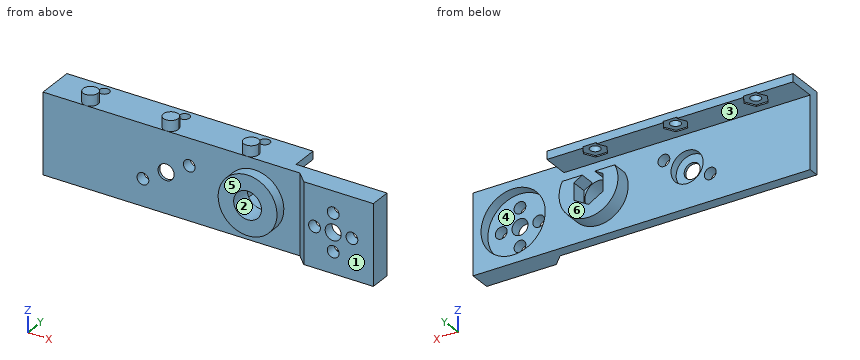
```python
from build123d import *

# Parameters (mm, degrees)
SKETCH_1_W          = 63
SKETCH_1_H          = 15
SKETCH_1_R          = 1.1
SKETCH_1_R_2        = 1.5
SKETCH_1_R_3        = 2.6
EXTRUDE_1_DEPTH     = 2
EXTRUDE_2_DEPTH     = 2
SKETCH_4_R          = 3
CUT_EXTRUDE_1_DEPTH = 1.5
SKETCH_5_W          = 46
SKETCH_5_H          = 1.5
EXTRUDE_3_DEPTH     = 5
SKETCH_2_3_R        = 0.95
CUT_EXTRUDE_2_DEPTH = 6
CUT_EXTRUDE_START   = -0.25
SKETCH_7_R          = 0.95
CUT_EXTRUDE_3_DEPTH = 0.25
SKETCH_1_3_W        = 15
SKETCH_1_3_H        = 15
SKETCH_1_3_R        = 6
SKETCH_1_3_R_2      = 1.5
SKETCH_1_3_R_3      = 1.1
EXTRUDE_4_DEPTH     = 2
EXTRUDE_START       = -2
SKETCH_1_4_W        = 15
SKETCH_1_4_H        = 15
SKETCH_1_4_R        = 6
SKETCH_1_4_R_2      = 1.5
SKETCH_1_4_R_3      = 1.1
EXTRUDE_5_DEPTH     = 2
SKETCH_1_5_R        = 6
CUT_EXTRUDE_4_DEPTH = 2
CUT_EXTRUDE_5_DEPTH = 15
SKETCH_9_R          = 5.5
SKETCH_9_R_2        = 2.6
EXTRUDE_6_DEPTH     = 3
CUT_EXTRUDE_START_2 = -3
CUT_EXTRUDE_6_DEPTH = 3
CUT_EXTRUDE_START_3 = -3.5
CUT_EXTRUDE_7_DEPTH = 3.5
EXTRUDE_START_2     = -4
SKETCH_9_2_R        = 5.5
SKETCH_9_2_R_2      = 2.6
EXTRUDE_7_DEPTH     = 4


with BuildPart() as part:
    # 草图1 → 凸台-拉伸1 (new body)
    with BuildSketch(Plane(origin=(0, 0, 0), x_dir=(1, 0, 0), z_dir=(0, 1, 0))):
        Rectangle(SKETCH_1_W, SKETCH_1_H)
        with Locations(Location((-4.169872981, -2.5, 0), (0, 0, 270))):
            Circle(SKETCH_1_R, mode=Mode.SUBTRACT)
        with Locations(Location((-8.5, 0, 0), (0, 0, 270))):
            Circle(SKETCH_1_R_2, mode=Mode.SUBTRACT)
        with Locations(Location((-12.830127019, 2.5, 0), (0, 0, 270))):
            Circle(SKETCH_1_R, mode=Mode.SUBTRACT)
        with Locations(Location((8, 0, 0), (0, 0, 270))):
            Circle(SKETCH_1_R_3, mode=Mode.SUBTRACT)
        with Locations(Location((24, 3.5, 0), (0, 0, 270))):
            Circle(SKETCH_1_R, mode=Mode.SUBTRACT)
        with Locations(Location((24, -3.5, 0), (0, 0, 270))):
            Circle(SKETCH_1_R, mode=Mode.SUBTRACT)
        with Locations(Location((20.5, 0, 0), (0, 0, 270))):
            Circle(SKETCH_1_R, mode=Mode.SUBTRACT)
        with Locations(Location((24, 0, 0), (0, 0, 270))):
            Circle(SKETCH_1_R_2, mode=Mode.SUBTRACT)
        with Locations(Location((27.5, 0, 0), (0, 0, 270))):
            Circle(SKETCH_1_R, mode=Mode.SUBTRACT)
    extrude(amount=EXTRUDE_1_DEPTH)

    # 草图2 → 凸台-拉伸2 (add)
    with BuildSketch(Plane.XY.offset(7.5)):
        with BuildLine():
            Line((-22.1, 1.4), (-24.9, 1.4))
            ThreePointArc((-24.9, 1.4), (-23.5, 0), (-22.1, 1.4))
        make_face()
        with BuildLine():
            ThreePointArc((-24.764911064, 2), (-24.865810289, 1.707509764), (-24.9, 1.4))
            Line((-24.9, 1.4), (-22.1, 1.4))
            ThreePointArc((-22.1, 1.4), (-22.134189711, 1.707509764), (-22.235088936, 2))
            Line((-22.235088936, 2), (-24.764911064, 2))
        make_face()
        with BuildLine():
            ThreePointArc((-22.235088936, 2), (-23.5, 2.8), (-24.764911064, 2))
            Line((-24.764911064, 2), (-22.235088936, 2))
        make_face()
        with BuildLine():
            Line((-7.1, 1.4), (-9.9, 1.4))
            ThreePointArc((-9.9, 1.4), (-8.5, 0), (-7.1, 1.4))
        make_face()
        with BuildLine():
            ThreePointArc((-9.764911064, 2), (-9.865810289, 1.707509764), (-9.9, 1.4))
            Line((-9.9, 1.4), (-7.1, 1.4))
            ThreePointArc((-7.1, 1.4), (-7.134189711, 1.707509764), (-7.235088936, 2))
            Line((-7.235088936, 2), (-9.764911064, 2))
        make_face()
        with BuildLine():
            ThreePointArc((-7.235088936, 2), (-8.5, 2.8), (-9.764911064, 2))
            Line((-9.764911064, 2), (-7.235088936, 2))
        make_face()
        with BuildLine():
            Line((7.9, 1.4), (5.1, 1.4))
            ThreePointArc((5.1, 1.4), (6.5, 0), (7.9, 1.4))
        make_face()
        with BuildLine():
            ThreePointArc((5.235088936, 2), (5.134189711, 1.707509764), (5.1, 1.4))
            Line((5.1, 1.4), (7.9, 1.4))
            ThreePointArc((7.9, 1.4), (7.865810289, 1.707509764), (7.764911064, 2))
            Line((7.764911064, 2), (5.235088936, 2))
        make_face()
        with BuildLine():
            ThreePointArc((7.764911064, 2), (6.5, 2.8), (5.235088936, 2))
            Line((5.235088936, 2), (7.764911064, 2))
        make_face()
    extrude(amount=EXTRUDE_2_DEPTH)

    # 草图4 → 切除-拉伸1 (cut)
    with BuildSketch(Plane(origin=(0, 2, 0), x_dir=(1, 0, 0), z_dir=(0, 1, 0))):
        with Locations(Location((-8.5, 0, 0), (0, 0, 270))):
            Circle(SKETCH_4_R)
    extrude(amount=-CUT_EXTRUDE_1_DEPTH, mode=Mode.SUBTRACT)

    # 草图5 → 凸台-拉伸3 (add)
    with BuildSketch(Plane(origin=(0, 2, 0), x_dir=(1, 0, 0), z_dir=(0, 1, 0))):
        with Locations((-8.5, -6.75)):
            Rectangle(SKETCH_5_W, SKETCH_5_H)
    extrude(amount=EXTRUDE_3_DEPTH)

    # 草图2<3> → 切除-拉伸2 (cut)
    with BuildSketch(Plane.XY.offset(7.5)):
        with Locations((-23.5, 5.4)):
            Circle(SKETCH_2_3_R)
        with Locations((-8.5, 5.4)):
            Circle(SKETCH_2_3_R)
        with Locations((6.5, 5.4)):
            Circle(SKETCH_2_3_R)
    extrude(amount=-CUT_EXTRUDE_2_DEPTH, mode=Mode.SUBTRACT)

    # 草图7 → 切除-拉伸3 (cut)
    # profile 1 of 3: a face of its own
    with BuildSketch(Plane(origin=(0, 0, 6), x_dir=(-1, 0, 0), z_dir=(0, 0, -1)).offset(CUT_EXTRUDE_START)):
        Polygon((-7.596965511, 3.5), (-5.403034489, 3.5), (-4.306068977, 5.4), (-5.403034489, 7.3), (-7.596965511, 7.3), (-8.693931023, 5.4), align=None)
        with Locations(Location((-6.5, 5.4, 0), (0, 0, 180))):
            Circle(SKETCH_7_R, mode=Mode.SUBTRACT)
    # profile 2 of 3: a face of its own
    with BuildSketch(Plane(origin=(0, 0, 6), x_dir=(-1, 0, 0), z_dir=(0, 0, -1)).offset(CUT_EXTRUDE_START)):
        Polygon((6.306068977, 5.4), (7.403034489, 3.5), (9.596965511, 3.5), (10.693931023, 5.4), (9.596965511, 7.3), (7.403034489, 7.3), align=None)
        with Locations(Location((8.5, 5.4, 0), (0, 0, 180))):
            Circle(SKETCH_7_R, mode=Mode.SUBTRACT)
    # profile 3 of 3: a face of its own
    with BuildSketch(Plane(origin=(0, 0, 6), x_dir=(-1, 0, 0), z_dir=(0, 0, -1)).offset(CUT_EXTRUDE_START)):
        Polygon((21.306068977, 5.4), (22.403034489, 3.5), (24.596965511, 3.5), (25.693931023, 5.4), (24.596965511, 7.3), (22.403034489, 7.3), align=None)
    extrude(amount=CUT_EXTRUDE_3_DEPTH, mode=Mode.SUBTRACT)

    # 草图1<3> → 凸台-拉伸4 (add)
    # profile 1 of 2: a face of its own
    with BuildSketch(Plane(origin=(0, 0, 0), x_dir=(1, 0, 0), z_dir=(0, 1, 0))):
        with Locations((24, 0)):
            Rectangle(SKETCH_1_3_W, SKETCH_1_3_H)
        with Locations((24, 0)):
            Circle(SKETCH_1_3_R, mode=Mode.SUBTRACT)
    # profile 2 of 2: a face of its own
    with BuildSketch(Plane(origin=(0, 0, 0), x_dir=(1, 0, 0), z_dir=(0, 1, 0))):
        with Locations((24, 0)):
            Circle(SKETCH_1_3_R)
        with Locations(Location((24, 0, 0), (0, 0, 270))):
            Circle(SKETCH_1_3_R_2, mode=Mode.SUBTRACT)
        with Locations(Location((27.5, 0, 0), (0, 0, 270))):
            Circle(SKETCH_1_3_R_3, mode=Mode.SUBTRACT)
        with Locations(Location((24, -3.5, 0), (0, 0, 270))):
            Circle(SKETCH_1_3_R_3, mode=Mode.SUBTRACT)
        with Locations(Location((20.5, 0, 0), (0, 0, 270))):
            Circle(SKETCH_1_3_R_3, mode=Mode.SUBTRACT)
        with Locations(Location((24, 3.5, 0), (0, 0, 270))):
            Circle(SKETCH_1_3_R_3, mode=Mode.SUBTRACT)
    extrude(amount=EXTRUDE_4_DEPTH)

    # 草图1<4> → 凸台-拉伸5 (add)
    # profile 1 of 2: a face of its own
    with BuildSketch(Plane(origin=(0, 0, 0), x_dir=(1, 0, 0), z_dir=(0, 1, 0)).offset(EXTRUDE_START)):
        with Locations((24, 0)):
            Rectangle(SKETCH_1_4_W, SKETCH_1_4_H)
        with Locations((24, 0)):
            Circle(SKETCH_1_4_R, mode=Mode.SUBTRACT)
    # profile 2 of 2: a face of its own
    with BuildSketch(Plane(origin=(0, 0, 0), x_dir=(1, 0, 0), z_dir=(0, 1, 0)).offset(EXTRUDE_START)):
        with Locations((24, 0)):
            Circle(SKETCH_1_4_R)
        with Locations(Location((24, 0, 0), (0, 0, 270))):
            Circle(SKETCH_1_4_R_2, mode=Mode.SUBTRACT)
        with Locations(Location((27.5, 0, 0), (0, 0, 270))):
            Circle(SKETCH_1_4_R_3, mode=Mode.SUBTRACT)
        with Locations(Location((24, -3.5, 0), (0, 0, 270))):
            Circle(SKETCH_1_4_R_3, mode=Mode.SUBTRACT)
        with Locations(Location((20.5, 0, 0), (0, 0, 270))):
            Circle(SKETCH_1_4_R_3, mode=Mode.SUBTRACT)
        with Locations(Location((24, 3.5, 0), (0, 0, 270))):
            Circle(SKETCH_1_4_R_3, mode=Mode.SUBTRACT)
    extrude(amount=EXTRUDE_5_DEPTH)

    # 草图1<5> → 切除-拉伸4 (cut)
    with BuildSketch(Plane(origin=(0, 0, 0), x_dir=(1, 0, 0), z_dir=(0, 1, 0))):
        with Locations(Location((24, 0, 0), (0, 0, 270))):
            Circle(SKETCH_1_5_R)
    extrude(amount=CUT_EXTRUDE_4_DEPTH, mode=Mode.SUBTRACT)

    # 草图8 → 切除-拉伸5 (cut)
    with BuildSketch(Plane(origin=(0, 0, -7.5), x_dir=(-1, 0, 0), z_dir=(0, 0, -1))):
        Polygon((-16.5, 0), (-18.5, -2), (-16.5, -2), align=None)
    extrude(amount=-CUT_EXTRUDE_5_DEPTH, mode=Mode.SUBTRACT)

    # 草图9 → 凸台-拉伸6 (add)
    with BuildSketch(Plane(origin=(0, 2, 0), x_dir=(1, 0, 0), z_dir=(0, 1, 0))):
        with Locations(Location((8, 0, 0), (0, 0, 270))):
            Circle(SKETCH_9_R)
        with Locations(Location((8, 0, 0), (0, 0, 270))):
            Circle(SKETCH_9_R_2, mode=Mode.SUBTRACT)
    extrude(amount=EXTRUDE_6_DEPTH)

    # 草图10 → 切除-拉伸6 (cut)
    with BuildSketch(Plane(origin=(0, 5, 0), x_dir=(1, 0, 0), z_dir=(0, 1, 0)).offset(CUT_EXTRUDE_START_2)):
        with BuildLine():
            Line((8, -3.175426481), (6.830127019, -2.5))
            Line((6.830127019, -2.5), (3.101020514, -2.5))
            ThreePointArc((3.101020514, -2.5), (8, -5.5), (12.898979486, -2.5))
            Line((12.898979486, -2.5), (9.169872981, -2.5))
            Line((9.169872981, -2.5), (8, -3.175426481))
        make_face()
        with BuildLine():
            Line((7.285857157, -2.5), (6.830127019, -2.5))
            Line((6.830127019, -2.5), (8, -3.175426481))
            Line((8, -3.175426481), (9.169872981, -2.5))
            Line((9.169872981, -2.5), (8.714142843, -2.5))
            ThreePointArc((8.714142843, -2.5), (8, -2.6), (7.285857157, -2.5))
        make_face()
    extrude(amount=CUT_EXTRUDE_6_DEPTH, mode=Mode.SUBTRACT)

    # 草图10<3> → 切除-拉伸7 (cut)
    with BuildSketch(Plane(origin=(0, 5, 0), x_dir=(1, 0, 0), z_dir=(0, 1, 0)).offset(CUT_EXTRUDE_START_3)):
        with BuildLine():
            Line((10.75, 1.58771324), (8, 3.175426481))
            Line((8, 3.175426481), (5.25, 1.58771324))
            Line((5.25, 1.58771324), (5.25, -1.58771324))
            Line((5.25, -1.58771324), (6.830127019, -2.5))
            Line((6.830127019, -2.5), (7.285857157, -2.5))
            ThreePointArc((7.285857157, -2.5), (6.43423683, 2.075665121), (10.6, 0))
            ThreePointArc((10.6, 0), (10.075665121, -1.56576317), (8.714142843, -2.5))
            Line((8.714142843, -2.5), (9.169872981, -2.5))
            Line((9.169872981, -2.5), (10.75, -1.58771324))
            Line((10.75, -1.58771324), (10.75, 1.58771324))
        make_face()
    extrude(amount=CUT_EXTRUDE_7_DEPTH, mode=Mode.SUBTRACT)

    # 草图9<2> → 凸台-拉伸7 (add)
    with BuildSketch(Plane(origin=(0, 2, 0), x_dir=(1, 0, 0), z_dir=(0, 1, 0)).offset(EXTRUDE_START_2)):
        with Locations(Location((8, 0, 0), (0, 0, 270))):
            Circle(SKETCH_9_2_R)
        with Locations(Location((8, 0, 0), (0, 0, 270))):
            Circle(SKETCH_9_2_R_2, mode=Mode.SUBTRACT)
    extrude(amount=EXTRUDE_7_DEPTH)


solid = part.part
```
Build history of the part. All positions in model axes, mm. Face numbers are marked on the shaded views. A direction names the side the tool comes from. Coordinates: 2 decimals unless noted, no trailing zeros. Write each loop counter-clockwise with the first axis right and the second up, starting at its lowest first coordinate (ties: lowest second). Pieces come first, ordered by that corner, then holes.
1. Drop flat-ended pins along their axis: pin 1 (2 mm diameter, centred on x = -1, z = 4.5, fed in from -Y); pin 2 (1.8 mm diameter, centred on x = -23.5, y = 6, fed in from -Z); pin 3 (1 mm diameter, centred on x = -3, z = -1, fed in from +Y). Give the stop position or say it passes through.
Answer block:
pin 1: stops at y = 0
pin 2: stops at z = 6.25
pin 3: stops at y = 2
2. Band-saw the part on C-C, the plane x = -0.5. Give the cut face in (y, z).
Answer block:
outline: (0, -7.5) - (2, -7.5) - (2, 6) - (7, 6) - (7, 7.5) - (0, 7.5) - close
3. 3-axis set-ups, long thin cutter, end or side, ignore diameter. For the marked faces 3, 4, 5 and 6: which of +Z, -Z, +X, -X, +Y, -Y reach the whole face in a straight line?
Answer block:
face 3: +X, -X, +Y
face 4: +Y
face 5: +Z, -Z, +X, -X, -Y
face 6: -Z, +X, -X, +Y
4. Band-saw the part on A-A, the plane x = 24. Give the cut face in (y, z), and give its area (3 significant figures).
Answer block:
outline: (-2, -7.5) - (2, -7.5) - (2, -6) - (0, -6) - (0, -4.6) - (-2, -4.6) - close; (-2, -2.4) - (0, -2.4) - (0, -1.5) - (-2, -1.5) - close; (-2, 1.5) - (0, 1.5) - (0, 2.4) - (-2, 2.4) - close; (-2, 4.6) - (0, 4.6) - (0, 6) - (2, 6) - (2, 7.5) - (-2, 7.5) - close
area: 21.2 mm2
5. Band-saw the part on B-B, the plane z = 0. Give the number of separate pieces and of enclosed holes in the cut face, and give its area (3 significant figures).
Answer block:
separate pieces: 6
enclosed holes: 0
area: 122 mm2
6. Drill centre lines: probe 1 along Z at (x, y) = (24, -0.35); probe 2 along X at (y, z) = (-1.15, 0); probe 3 along X at (y, z) = (-0.75, -3). Where is each one in solid material? Low to high.
Answer block:
probe 1: z = -7.5 to -4.6, -2.4 to -1.5, 1.5 to 2.4, 4.6 to 7.5
probe 2: x = 2.5 to 5.4, 10.6 to 13.5, 17.65 to 19.4, 21.6 to 22.5, 25.5 to 26.4, 28.6 to 31.5
probe 3: x = 3.39 to 12.61, 17.25 to 23.02, 24.98 to 31.5
7. Pull direction X, two halves, no side cores. Call the marked faces 1 and 2: released by +X, released by -X, zero draft, split by the parting line, or undercut.
Answer block:
face 1: zero draft
face 2: undercut
